```python
from build123d import *

# Parameters (mm, degrees)
SKETCH_1_W          = 140
SKETCH_1_H          = 70
EXTRUDE_1_DEPTH     = 6
SKETCH_2_R          = 15
EXTRUDE_2_DEPTH     = 10
SKETCH_5_R          = 5
EXTRUDE_4_DEPTH     = 15
SKETCH_7_W          = 5
SKETCH_7_H          = 49
CUT_EXTRUDE_1_DEPTH = 6
EXTRUDE_5_DEPTH     = 30
EXTRUDE_START       = -30
EXTRUDE_6_DEPTH     = 30


with BuildPart() as part:
    # 草图1 → 凸台-拉伸1 (new body)
    with BuildSketch(Plane(origin=(0, 0, 0), x_dir=(1, 0, 0), z_dir=(0, 1, 0))):
        with Locations((3.730042991, 0.147818203)):
            Rectangle(SKETCH_1_W, SKETCH_1_H)
    extrude(amount=EXTRUDE_1_DEPTH)

    # 草图2 → 凸台-拉伸2 (add)
    with BuildSketch(Plane(origin=(0, 6, 0), x_dir=(1, 0, 0), z_dir=(0, 1, 0))):
        with Locations(Location((3.730042991, 0.147818203, 0), (0, 0, 270))):
            Circle(SKETCH_2_R)
    extrude(amount=EXTRUDE_2_DEPTH)

    # 草图5 → 凸台-拉伸4 (add)
    with BuildSketch(Plane(origin=(0, 16, 0), x_dir=(1, 0, 0), z_dir=(0, 1, 0))):
        with Locations(Location((3.730042991, 0.147818203, 0), (0, 0, 270))):
            Circle(SKETCH_5_R)
    extrude(amount=EXTRUDE_4_DEPTH)

    # 草图6 → 旋转2 (revolve)
    with BuildSketch(Plane(origin=(0, 31, 0), x_dir=(1, 0, 0), z_dir=(0, 1, 0))):
        with BuildLine():
            Line((3.730042991, 10.047818203), (3.730042991, -9.752181797))
            ThreePointArc((3.730042991, -9.752181797), (13.630042991, 0.147818203), (3.730042991, 10.047818203))
        make_face()
    revolve(axis=Axis((3.730042991, 31, -10.047818203), (0, 0, 1)))

    # 草图7 → 切除-拉伸1 (cut)
    with BuildSketch(Plane.XZ):
        with Locations((25.230042991, -0.380891395)):
            Rectangle(SKETCH_7_W, SKETCH_7_H)
        with Locations((-37.769957009, -0.380891395)):
            Rectangle(SKETCH_7_W, SKETCH_7_H)
        with Locations((35.230042991, -0.380891395)):
            Rectangle(SKETCH_7_W, SKETCH_7_H)
        with Locations((45.230042991, -0.380891395)):
            Rectangle(SKETCH_7_W, SKETCH_7_H)
        with Locations((-27.769957009, -0.380891395)):
            Rectangle(SKETCH_7_W, SKETCH_7_H)
        with Locations((-17.769957009, -0.380891395)):
            Rectangle(SKETCH_7_W, SKETCH_7_H)
    extrude(amount=-CUT_EXTRUDE_1_DEPTH, mode=Mode.SUBTRACT)

    # 草图9 → 凸台-拉伸5 (add)
    with BuildSketch(Plane.ZY.offset(66.269957009)):
        with BuildLine():
            Line((29.852181797, 6), (34.852181797, 6))
            ThreePointArc((34.852181797, 6), (32.352181797, 8.5), (29.852181797, 6))
        make_face()
        with BuildLine():
            Line((-35.147818203, 6), (-30.147818203, 6))
            ThreePointArc((-30.147818203, 6), (-32.647818203, 8.5), (-35.147818203, 6))
        make_face()
        with BuildLine():
            Line((21.852181797, 6), (24.852181797, 6))
            ThreePointArc((24.852181797, 6), (23.352181797, 7.5), (21.852181797, 6))
        make_face()
        with BuildLine():
            Line((-25.147818203, 6), (-22.147818203, 6))
            ThreePointArc((-22.147818203, 6), (-23.647818203, 7.5), (-25.147818203, 6))
        make_face()
    extrude(amount=-EXTRUDE_5_DEPTH)

    # 草图11 → 凸台-拉伸6 (add)
    with BuildSketch(Plane(origin=(73.730042991, 0, 0), x_dir=(0, 0, -1), z_dir=(1, 0, 0)).offset(EXTRUDE_START)):
        with BuildLine():
            Line((30.147818203, 6), (35.147818203, 6))
            ThreePointArc((35.147818203, 6), (32.647818203, 8.5), (30.147818203, 6))
        make_face()
        with BuildLine():
            Line((-34.852181797, 6), (-29.852181797, 6))
            ThreePointArc((-29.852181797, 6), (-32.352181797, 8.5), (-34.852181797, 6))
        make_face()
        with BuildLine():
            Line((22.147818203, 6), (25.147818203, 6))
            ThreePointArc((25.147818203, 6), (23.647818203, 7.5), (22.147818203, 6))
        make_face()
        with BuildLine():
            Line((-24.852181797, 6), (-21.852181797, 6))
            ThreePointArc((-21.852181797, 6), (-23.352181797, 7.5), (-24.852181797, 6))
        make_face()
    extrude(amount=EXTRUDE_6_DEPTH)


solid = part.part
```
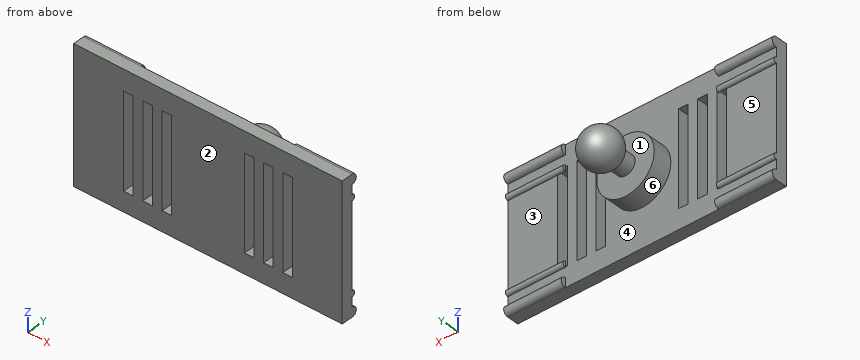
Build history of the part. All positions in model axes, mm. Face numbers are marked on the shaded views. A direction names the side the tool comes from. Round coordinates to 2 decimals unless told otherwise and drop trailing zeros. Order: outer loops, then holes, each group sorted by start corner. A loop starts at its lowest first (then second) coordinate and runs counter-clockwise, first axis right, second up. Notation, with made-up numbers: (23, 61.5) - (49, 61.5) arc R21 cw to (49, 76.5) - close; hole circle Ø6 at (-2.5, -1). An arc over 180 degrees is marked (long way). Use a Markdown table: item, result.
1) Saw through at D-D on z = 28. Write the cut outline in (x, y), and give its area (3 significant figures).
Recorded:
| item | result |
|---|---|
| outline | (-66.27, 0) - (73.73, 0) - (73.73, 6) - (-66.27, 6) - close |
| area | 840 mm² |
2) Flat gauge pins, fed straight in: pin 1 Ø10 at (x, z) = (-51, -13.5) entering from -Y; pin 2 Ø1 at (y, z) = (22.5, 7.5) entering from -X; pin 3 Ø3 at (x, z) = (3, -17) entering from +Y; pin 4 Ø4 at (y, z) = (29, -0.5) entering from -X. Where does each tip first touch, or does it go through?
Recorded:
| item | result |
|---|---|
| pin 1 | stops at y = 0 |
| pin 2 | passes through |
| pin 3 | stops at y = 6 |
| pin 4 | stops at x = -6.17 |
3) Saw through at A-A on z = -17. Write the cut outline in (x, y), and give its area (3 significant figures).
Recorded:
| item | result |
|---|---|
| outline | (-66.27, 0) - (-40.27, 0) - (-40.27, 6) - (-66.27, 6) - close; (-35.27, 0) - (-30.27, 0) - (-30.27, 6) - (-35.27, 6) - close; (-25.27, 0) - (-20.27, 0) - (-20.27, 6) - (-25.27, 6) - close; (-15.27, 0) - (22.73, 0) - (22.73, 6) - (-15.27, 6) - close; (27.73, 0) - (32.73, 0) - (32.73, 6) - (27.73, 6) - close; (37.73, 0) - (42.73, 0) - (42.73, 6) - (37.73, 6) - close; (47.73, 0) - (73.73, 0) - (73.73, 6) - (47.73, 6) - close |
| area | 660 mm² |
4) Saw through at B-B on x = 15. Write the cut outline in (y, z).
Recorded:
| item | result |
|---|---|
| outline | (0, -35.15) - (6, -35.15) - (6, -10.05) - (16, -10.05) - (16, 9.75) - (6, 9.75) - (6, 34.85) - (0, 34.85) - close |
5) Wall check: L1, parallel to Y at x = 0, z = 19; L2, parallel to Z at x = 3, y = 31; L3, parallel to Z at x = 3, y = 8. Give the ranges that are in metal, low to high.
Recorded:
| item | result |
|---|---|
| L1 | y = 0 to 6 |
| L2 | z = -10.02 to 9.73 |
| L3 | z = -15.13 to 14.83 |
6) Pull direction X, two halves, no side cores. Call the marked faces 4, 5 and 6: pulls with the +X half, pulls with the -X half, needs draft (parallel to the pull), parting line crosses it, or undercut.
Recorded:
| item | result |
|---|---|
| face 4 | undercut |
| face 5 | needs draft |
| face 6 | parting line crosses it |
7) Saw through at C-C on y = 17.5. Write the cut outline in (x, z), and give its area (3 significant figures).
Recorded:
| item | result |
|---|---|
| outline | circle Ø10 at (3.73, -0.15) |
| area | 78.5 mm² |
8) Tool access for the marked faces 1, 2 and 3: list every direction of +Z, -Z, +X, -X, +Y, -Y with a clear straight run to the whole face (end or side of a thin tool).
Recorded:
| item | result |
|---|---|
| face 1 | none |
| face 2 | +Z, -Z, +X, -X, -Y |
| face 3 | +X, +Y |
